Source: CAD feature listing. Evaluate the final solid. Frame: model axes, mm. A direction names the side the tool comes from. Give positions to 0.01 mm unless a question says otherwise; leave off trailing zeros. Loops run counter-clockwise (first coordinate to the right, second up) from the corner with the lowest first, then second, coordinate; pieces in that order, holes last. Notation, with made-up numbers: M -28.5,55.5 L -9.5,55.5 A24 cw -9.5,73.5 Z; hole C -38,-27.5 d9. An arc over 180 degrees is marked long. Answer in a Markdown table with one row per item.
```python
from build123d import *

# Parameters (mm, degrees)
SKETCH1_R           = 2
BOSS_EXTRUDE1_DEPTH = 15.24
BOSS_EXTRUDE2_START = -31.75
SKETCH1_3_R         = 3.175
SKETCH1_3_R_2       = 2
BOSS_EXTRUDE2_DEPTH = 31.75
SKETCH2_R           = 6.35
BOSS_EXTRUDE3_DEPTH = 3.175


with BuildPart() as part:
    # Sketch1 → Boss-Extrude1 (new body)
    with BuildSketch(Plane(origin=(0, 0, 0), x_dir=(0, 0, -1), z_dir=(1, 0, 0))):
        with Locations(Location((0, 0, 0), (0, 0, 180))):
            Circle(SKETCH1_R)
    extrude(amount=BOSS_EXTRUDE1_DEPTH)

    # Sketch1_3 → Boss-Extrude2 (add)
    with BuildSketch(Plane(origin=(0, 0, 0), x_dir=(0, 0, -1), z_dir=(1, 0, 0)).offset(BOSS_EXTRUDE2_START)):
        Circle(SKETCH1_3_R)
        with Locations(Location((0, 0, 0), (0, 0, 180))):
            Circle(SKETCH1_3_R_2)
    extrude(amount=BOSS_EXTRUDE2_DEPTH)

    # Sketch2 → Boss-Extrude3 (add)
    with BuildSketch(Plane.ZY.offset(31.75)):
        Circle(SKETCH2_R)
    extrude(amount=BOSS_EXTRUDE3_DEPTH)


solid = part.part
```
Q1. Ray query, probe 1 along X at (y, z) = (-2.25, -4.75) (3 decimals); probe 2 along Y at (x, z) = (2, 0.75); probe 3 along Z at (x, y) = (-20, 1.75). Return the intervals inside material, ascending. Write a range as from..to.
Values follow:
| item | result |
|---|---|
| probe 1 | -34.925..-31.75 |
| probe 2 | -1.85..1.85 |
| probe 3 | -2.65..2.65 |
Q2. Section query A-A (y = 0). Output: boundary loops of the cut face in (x, z) (3 decimals).
Values follow:
| item | result |
|---|---|
| outline | M -34.925,-6.35 L -31.75,-6.35 L -31.75,-3.175 L 0,-3.175 L 0,-2 L 15.24,-2 L 15.24,2 L 0,2 L 0,3.175 L -31.75,3.175 L -31.75,6.35 L -34.925,6.35 Z |
Q3. Section query C-C (x = -30). Output: boundary loops of the cut face in (y, z) (3 decimals), plus the area to 3 significant figures.
Values follow:
| item | result |
|---|---|
| outline | C 0,0 d6.35 |
| area | 31.7 mm^2 |
Q4. Reachability of faces 1 (the flat face through (-34.925, 0, 0)), 2 (the flat face through (-31.75, 3, -2)) from +Z, -Z, +X, -X, +Y, -Y: full face, straight path, thin tool, end or side. Return the list, or none.
Values follow:
| item | result |
|---|---|
| face 1 | +Z, -Z, -X, +Y, -Y |
| face 2 | +X |
Q5. Section query D-D (z = 2.5). Output: boundary loops of the cut face in (x, y) (3 decimals).
Values follow:
| item | result |
|---|---|
| outline | M -34.925,-5.837 L -31.75,-5.837 L -31.75,-1.957 L 0,-1.957 L 0,1.957 L -31.75,1.957 L -31.75,5.837 L -34.925,5.837 Z |
Q6. Section query B-B (z = 0.25). Output: boundary loops of the cut face in (x, y) (3 decimals).
Values follow:
| item | result |
|---|---|
| outline | M -34.925,-6.345 L -31.75,-6.345 L -31.75,-3.165 L 0,-3.165 L 0,-1.984 L 15.24,-1.984 L 15.24,1.984 L 0,1.984 L 0,3.165 L -31.75,3.165 L -31.75,6.345 L -34.925,6.345 Z |
Q7. Contact query for flat-ended pins moving along their axis: pin 1 Ø2 at (x, z) = (-20, -1) entering from -Y (3 decimals); pin 2 Ø4 at (x, y) = (0, -2) entering from -Z (3 decimals); pin 3 Ø1 at (x, y) = (-5.5, 2) entering from -Z; pin 4 Ø4 at (y, z) = (-2, -1.5) entering from +X. Output: stop coordinate, or through.
Values follow:
| item | result |
|---|---|
| pin 1 | y = -3.175 |
| pin 2 | z = -3.175 |
| pin 3 | z = -2.8 |
| pin 4 | x = 15.24 |
